CAD build for the part. Positions are in the model's coordinates, mm. A direction names the side the tool comes from. Give positions to 0.01 mm unless a question says otherwise; leave off trailing zeros. Loops run counter-clockwise (first coordinate to the right, second up) from the corner with the lowest first, then second, coordinate; pieces in that order, holes last. Notation, with made-up numbers: M -12.75,-0.75 L 42.25,-0.75 A23 ccw 42.25,13.25 Z; hole C 8.5,80.25 d3. An arc over 180 degrees is marked long. One line per question, with ' | ' between items.
```python
from build123d import *

# Parameters (mm, degrees)
SKETCH1_W           = 200
SKETCH1_H           = 194
BOSS_EXTRUDE2_DEPTH = 10
SKETCH2_R           = 1.1
CUT_EXTRUDE1_DEPTH  = 5
SKETCH5_R           = 1.65
CUT_EXTRUDE3_DEPTH  = 284.051232112
CUT_EXTRUDE4_DEPTH  = 10


with BuildPart() as part:
    # Sketch1 → Boss-Extrude2 (new body)
    with BuildSketch(Plane(origin=(0, 0, 0), x_dir=(1, 0, 0), z_dir=(0, 1, 0))):
        with Locations((103, 100)):
            Rectangle(SKETCH1_W, SKETCH1_H)
    extrude(amount=BOSS_EXTRUDE2_DEPTH)

    # Sketch2 → Cut-Extrude1 (cut)
    with BuildSketch(Plane(origin=(0, 10, 0), x_dir=(1, 0, 0), z_dir=(0, 1, 0))):
        with Locations(Location((115.5, 187.5, 0), (0, 0, 270))):
            Circle(SKETCH2_R)
        with Locations(Location((140.5, 187.5, 0), (0, 0, 270))):
            Circle(SKETCH2_R)
        with Locations(Location((165.5, 187.5, 0), (0, 0, 270))):
            Circle(SKETCH2_R)
        with Locations(Location((190.5, 187.5, 0), (0, 0, 270))):
            Circle(SKETCH2_R)
        with Locations(Location((115.5, 162.5, 0), (0, 0, 270))):
            Circle(SKETCH2_R)
        with Locations(Location((140.5, 162.5, 0), (0, 0, 270))):
            Circle(SKETCH2_R)
        with Locations(Location((165.5, 162.5, 0), (0, 0, 270))):
            Circle(SKETCH2_R)
        with Locations(Location((190.5, 162.5, 0), (0, 0, 270))):
            Circle(SKETCH2_R)
        with Locations(Location((115.5, 137.5, 0), (0, 0, 270))):
            Circle(SKETCH2_R)
        with Locations(Location((140.5, 137.5, 0), (0, 0, 270))):
            Circle(SKETCH2_R)
        with Locations(Location((165.5, 137.5, 0), (0, 0, 270))):
            Circle(SKETCH2_R)
        with Locations(Location((190.5, 137.5, 0), (0, 0, 270))):
            Circle(SKETCH2_R)
        with Locations(Location((115.5, 112.5, 0), (0, 0, 270))):
            Circle(SKETCH2_R)
        with Locations(Location((140.5, 112.5, 0), (0, 0, 270))):
            Circle(SKETCH2_R)
        with Locations(Location((165.5, 112.5, 0), (0, 0, 270))):
            Circle(SKETCH2_R)
        with Locations(Location((190.5, 112.5, 0), (0, 0, 270))):
            Circle(SKETCH2_R)
        with Locations(Location((65.5, 112.5, 0), (0, 0, 90))):
            Circle(SKETCH2_R)
        with Locations(Location((90.5, 112.5, 0), (0, 0, 90))):
            Circle(SKETCH2_R)
        with Locations(Location((40.5, 112.5, 0), (0, 0, 90))):
            Circle(SKETCH2_R)
        with Locations(Location((15.5, 112.5, 0), (0, 0, 90))):
            Circle(SKETCH2_R)
        with Locations(Location((15.5, 137.5, 0), (0, 0, 90))):
            Circle(SKETCH2_R)
        with Locations(Location((40.5, 137.5, 0), (0, 0, 90))):
            Circle(SKETCH2_R)
        with Locations(Location((65.5, 137.5, 0), (0, 0, 90))):
            Circle(SKETCH2_R)
        with Locations(Location((90.5, 137.5, 0), (0, 0, 90))):
            Circle(SKETCH2_R)
        with Locations(Location((65.5, 162.5, 0), (0, 0, 90))):
            Circle(SKETCH2_R)
        with Locations(Location((90.5, 162.5, 0), (0, 0, 90))):
            Circle(SKETCH2_R)
        with Locations(Location((40.5, 162.5, 0), (0, 0, 90))):
            Circle(SKETCH2_R)
        with Locations(Location((15.5, 162.5, 0), (0, 0, 90))):
            Circle(SKETCH2_R)
        with Locations(Location((15.5, 187.5, 0), (0, 0, 90))):
            Circle(SKETCH2_R)
        with Locations(Location((40.5, 187.5, 0), (0, 0, 90))):
            Circle(SKETCH2_R)
        with Locations(Location((65.5, 187.5, 0), (0, 0, 90))):
            Circle(SKETCH2_R)
        with Locations(Location((90.5, 187.5, 0), (0, 0, 90))):
            Circle(SKETCH2_R)
        with Locations(Location((190.5, 87.5, 0), (0, 0, 90))):
            Circle(SKETCH2_R)
        with Locations(Location((165.5, 87.5, 0), (0, 0, 90))):
            Circle(SKETCH2_R)
        with Locations(Location((140.5, 87.5, 0), (0, 0, 90))):
            Circle(SKETCH2_R)
        with Locations(Location((115.5, 87.5, 0), (0, 0, 90))):
            Circle(SKETCH2_R)
        with Locations(Location((190.5, 62.5, 0), (0, 0, 90))):
            Circle(SKETCH2_R)
        with Locations(Location((165.5, 62.5, 0), (0, 0, 90))):
            Circle(SKETCH2_R)
        with Locations(Location((140.5, 62.5, 0), (0, 0, 90))):
            Circle(SKETCH2_R)
        with Locations(Location((115.5, 62.5, 0), (0, 0, 90))):
            Circle(SKETCH2_R)
        with Locations(Location((190.5, 37.5, 0), (0, 0, 90))):
            Circle(SKETCH2_R)
        with Locations(Location((165.5, 37.5, 0), (0, 0, 90))):
            Circle(SKETCH2_R)
        with Locations(Location((140.5, 37.5, 0), (0, 0, 90))):
            Circle(SKETCH2_R)
        with Locations(Location((115.5, 37.5, 0), (0, 0, 90))):
            Circle(SKETCH2_R)
        with Locations(Location((190.5, 12.5, 0), (0, 0, 90))):
            Circle(SKETCH2_R)
        with Locations(Location((165.5, 12.5, 0), (0, 0, 90))):
            Circle(SKETCH2_R)
        with Locations(Location((140.5, 12.5, 0), (0, 0, 90))):
            Circle(SKETCH2_R)
        with Locations(Location((115.5, 12.5, 0), (0, 0, 90))):
            Circle(SKETCH2_R)
        with Locations(Location((90.5, 12.5, 0), (0, 0, 270))):
            Circle(SKETCH2_R)
        with Locations(Location((65.5, 12.5, 0), (0, 0, 270))):
            Circle(SKETCH2_R)
        with Locations(Location((40.5, 12.5, 0), (0, 0, 270))):
            Circle(SKETCH2_R)
        with Locations(Location((15.5, 12.5, 0), (0, 0, 270))):
            Circle(SKETCH2_R)
        with Locations(Location((90.5, 37.5, 0), (0, 0, 270))):
            Circle(SKETCH2_R)
        with Locations(Location((65.5, 37.5, 0), (0, 0, 270))):
            Circle(SKETCH2_R)
        with Locations(Location((40.5, 37.5, 0), (0, 0, 270))):
            Circle(SKETCH2_R)
        with Locations(Location((15.5, 37.5, 0), (0, 0, 270))):
            Circle(SKETCH2_R)
        with Locations(Location((90.5, 62.5, 0), (0, 0, 270))):
            Circle(SKETCH2_R)
        with Locations(Location((65.5, 62.5, 0), (0, 0, 270))):
            Circle(SKETCH2_R)
        with Locations(Location((40.5, 62.5, 0), (0, 0, 270))):
            Circle(SKETCH2_R)
        with Locations(Location((15.5, 62.5, 0), (0, 0, 270))):
            Circle(SKETCH2_R)
        with Locations(Location((90.5, 87.5, 0), (0, 0, 270))):
            Circle(SKETCH2_R)
        with Locations(Location((65.5, 87.5, 0), (0, 0, 270))):
            Circle(SKETCH2_R)
        with Locations(Location((40.5, 87.5, 0), (0, 0, 270))):
            Circle(SKETCH2_R)
        with Locations(Location((15.5, 87.5, 0), (0, 0, 270))):
            Circle(SKETCH2_R)
    extrude(amount=-CUT_EXTRUDE1_DEPTH, mode=Mode.SUBTRACT)

    # Sketch5 → Cut-Extrude3 (cut, through all)
    with BuildSketch(Plane(origin=(0, 10, 0), x_dir=(1, 0, 0), z_dir=(0, 1, 0))):
        with Locations(Location((15.5, 193, 0), (0, 0, 270))):
            Circle(SKETCH5_R)
        with Locations(Location((65.5, 193, 0), (0, 0, 270))):
            Circle(SKETCH5_R)
        with Locations(Location((140.5, 193, 0), (0, 0, 270))):
            Circle(SKETCH5_R)
        with Locations(Location((190.5, 193, 0), (0, 0, 270))):
            Circle(SKETCH5_R)
        with Locations(Location((190.5, 7, 0), (0, 0, 90))):
            Circle(SKETCH5_R)
        with Locations(Location((140.5, 7, 0), (0, 0, 90))):
            Circle(SKETCH5_R)
        with Locations(Location((65.5, 7, 0), (0, 0, 90))):
            Circle(SKETCH5_R)
        with Locations(Location((15.5, 7, 0), (0, 0, 90))):
            Circle(SKETCH5_R)
    extrude(amount=-CUT_EXTRUDE3_DEPTH, mode=Mode.SUBTRACT)

    # Sketch6 → Cut-Extrude4 (cut)
    with BuildSketch(Plane(origin=(0, 10, 0), x_dir=(1, 0, 0), z_dir=(0, 1, 0))):
        with BuildLine():
            Line((48, 33), (48, 167))
            ThreePointArc((48, 167), (53, 172), (58, 167))
            Line((58, 167), (58, 33))
            ThreePointArc((58, 33), (53, 28), (48, 33))
        make_face()
        with BuildLine():
            Line((158, 33), (158, 167))
            ThreePointArc((158, 167), (153, 172), (148, 167))
            Line((148, 167), (148, 33))
            ThreePointArc((148, 33), (153, 28), (158, 33))
        make_face()
    extrude(amount=-CUT_EXTRUDE4_DEPTH, mode=Mode.SUBTRACT)


solid = part.part
```
Item 1: Mould opens along Z. For faces 1 (the flat face through (148, 5, -101)), 2 (the flat face through (102, 5, -197)), 3 (the flat face through (102, 0, -101)) say: pulls with the +Z half, pulls with the -Z half, needs draft (parallel to the pull), parting line crosses it, or undercut.
Conclusion:
face 1: undercut | face 2: pulls with the -Z half | face 3: needs draft
Item 2: Drill centre lines: line 1 along X through (y, z) = (0.5, -157); line 2 along X through (y, z) = (5, -193); line 3 along Z through (x, y) = (141, 0.5). Where is each one in solid material? Low to high. Write a range as [from, to].
Conclusion:
line 1: [3, 48], [58, 148], [158, 203] | line 2: [3, 13.85], [17.15, 63.85], [67.15, 138.85], [142.15, 188.85], [192.15, 203] | line 3: [-197, -194.57], [-191.43, -8.57], [-5.43, -3]
Item 3: Drop a flat-ended pin along its axis: P1, Ø1.8, axis at x = 140.5, z = -162.5, coming from the +Y side. Give the stop position or say it passes through.
Conclusion:
P1: y = 5
Item 4: Saw through at B-B on z = -157.5. Give the cut face in (x, y).
Conclusion:
outline: M 3,0 L 48,0 L 48,10 L 3,10 Z; M 58,0 L 148,0 L 148,10 L 58,10 Z; M 158,0 L 203,0 L 203,10 L 158,10 Z
Item 5: 3-axis set-ups, long thin cutter, end or side, ignore diameter. For faces 4 (the cylindrical face through (53, 5, -172)), 5 (the flat face through (102, 5, -3)): which of +Z, -Z, +X, -X, +Y, -Y reach the whole face in a straight line?
Conclusion:
face 4: +Y, -Y | face 5: +Z, +X, -X, +Y, -Y
Item 6: Saw through at C-C on x = 153. Give the cut face in (y, z), and give its area (3 significant figures).
Conclusion:
outline: M 0,-197 L 10,-197 L 10,-172 L 0,-172 Z; M 0,-28 L 10,-28 L 10,-3 L 0,-3 Z | area: 500 mm²
Item 7: Saw through at A-A on y = 3. State how many separate pieces and enclosed holes the cut face has, and give its area (3 significant figures).
Conclusion:
separate pieces: 1 | enclosed holes: 10 | area: 35,900 mm²
